from build123d import *

# Parameters (mm, degrees)
BOSS_EXTRUDE1_DEPTH = 80
SKETCH2_R           = 15
CUT_EXTRUDE1_DEPTH  = 35
CUT_EXTRUDE2_START  = 35
SKETCH3_R           = 9.75
CUT_EXTRUDE2_DEPTH  = 120


with BuildPart() as part:
    # Sketch1 → Boss-Extrude1 (new body)
    with BuildSketch(Plane.XY):
        Polygon((80, 80), (80, -80), (-80, 80), align=None)
    extrude(amount=BOSS_EXTRUDE1_DEPTH)

    # Sketch2 → Cut-Extrude1 (cut)
    with BuildSketch(Plane(origin=(0, 80, 0), x_dir=(1, 0, 0), z_dir=(0, 1, 0))):
        with Locations(Location((57, -39.75, 0), (0, 0, 270))):
            Circle(SKETCH2_R)
    extrude(amount=-CUT_EXTRUDE1_DEPTH, mode=Mode.SUBTRACT)

    # Sketch3 → Cut-Extrude2 (cut)
    with BuildSketch(Plane(origin=(0, 45, 0), x_dir=(1, 0, 0), z_dir=(0, 1, 0)).offset(CUT_EXTRUDE2_START)):
        with Locations(Location((57, -39.75, 0), (0, 0, 270))):
            Circle(SKETCH3_R)
    extrude(amount=-CUT_EXTRUDE2_DEPTH, mode=Mode.SUBTRACT)


solid = part.part
Here's how the part is built. I have some questions about the finished solid (model axes, mm). A direction names the side the tool comes from. Coordinates: 2 decimals unless noted, no trailing zeros. Write each loop counter-clockwise with the first axis right and the second up, starting at its lowest first coordinate (ties: lowest second). Pieces come first, ordered by that corner, then holes.
1) I'm going to push flat-ended pins straight in: pin 1 (3 mm diameter, centred on x = -23.5, z = 45.5, fed in from -Y); pin 2 (6 mm diameter, centred on x = -28.5, z = 30, fed in from -Y); pin 3 (21.5 mm diameter, centred on x = 57.5, z = 39, fed in from +Y). Where does each tip first touch, or does it pass through?
Filled in:
pin 1: stops at y = 22
pin 2: stops at y = 25.5
pin 3: stops at y = 45
2) Thinking about a two-plate mould opening in X: for faces 1 (the face through (19, 19, 80)), 2 (the face through (63.59, 3.095, 32.564)), 3 (the face through (1, -1, 39)), which applies, +X half, -X half, draft (parallel to the pull), parting line (faces both ways), or undercut?
Filled in:
face 1: draft
face 2: undercut
face 3: -X half
3) If we section it at C-C (z = 39.75): List the corners of the cut face in (x, y) for me, plus the area to 3 significant figures.
Filled in:
outline: (-80, 80) - (80, -80) - (80, 80) - (72, 80) - (72, 45) - (66.75, 45) - (66.75, -40) - (47.25, -40) - (47.25, 45) - (42, 45) - (42, 80) - close
area: 10,100 mm2
4) If we section it at B-B (x = 55): List the corners of the cut face in (y, z) for me, plus the area to 3 significant figures.
Filled in:
outline: (-55, 0) - (80, 0) - (80, 24.88) - (45, 24.88) - (45, 30.21) - (-40, 30.21) - (-40, 49.29) - (45, 49.29) - (45, 54.62) - (80, 54.62) - (80, 80) - (-55, 80) - close
area: 8,140 mm2
5) If we section it at D-D (y = 13): List the corners of the cut face in (x, z) for me.
Filled in:
outline: (-13, 0) - (80, 0) - (80, 80) - (-13, 80) - close; hole circle Ø19.5 at (57, 39.75)
6) Which directions (+Z, -Z, +X, -X, +Y, -Y) give clear straight access to the entire face, cutting with the end or side of a thin tool? Please do faces 4 (the face through (-1, 80, 39)), 5 (the face through (47.87, 62.74, 27.85)).
Filled in:
face 4: +Z, -Z, +X, -X, +Y
face 5: +Y
7) If I drill on line 1 (X direction, y = 63, z = 39.75); line 2 (X direction, y = 62, z = 39); line 3 (Z direction, x = 61, y = -33), over which ranges is the centre line in solid material (lowest first)?
Filled in:
line 1: x = -63 to 42, 72 to 80
line 2: x = -62 to 42.02, 71.98 to 80
line 3: z = 0 to 30.86, 48.64 to 80
8) If we section it at A-A (y = -31.5): List the corners of the cut face in (x, z) for me, plus the area to 3 significant figures.
Filled in:
outline: (31.5, 0) - (80, 0) - (80, 80) - (31.5, 80) - close; hole circle Ø19.5 at (57, 39.75)
area: 3,580 mm2
